Check sheet for the modelled part. Datum: model origin and axes. Units: mm. Round coordinates to 2 decimals unless told otherwise and drop trailing zeros. Order: outer loops, then holes, each group sorted by start corner. A loop starts at its lowest first (then second) coordinate and runs counter-clockwise, first axis right, second up. Notation, with made-up numbers: (-17, 42.5) -> (37, 42.5) arc R17 cw to (37, 65.5) -> close; hole circle Ø9 at (7, 5). An arc over 180 degrees is marked (long way). Answer in a Markdown table with one row per item. Add a question column.
1. Depth check by flat-ended pin: P1, Ø1.9, axis at x = 1, z = 76.5, coming from the -Y side. Enter the tip coordinate at first touch or a pass-through.
2. Sectioned sample at D-D, the plane z = 27. Record the boundary of the cut face in (x, y).
3. Sectioned sample at B-B, the plane x = 24.8. Record the boundary of the cut face in (y, z), then the cut area to 3 significant figures.
4. Sectioned sample at A-A, the plane z = 0. Record the boundary of the cut face in (x, y), then the cut area to 3 significant figures.
5. Sectioned sample at C-C, the plane y = 3. Count the separate pieces of the cut face and the enclosed holes in it, then the cut area to 3 significant figures.
6. Material ranges on L1, parallel to Z at x = 0, y = 2.6; L2, parallel to X at y = 1.15, z = 24.8; L3, parallel to Y at x = 22.5, z = 75.5, recorded low to high. Write a range as from..to.
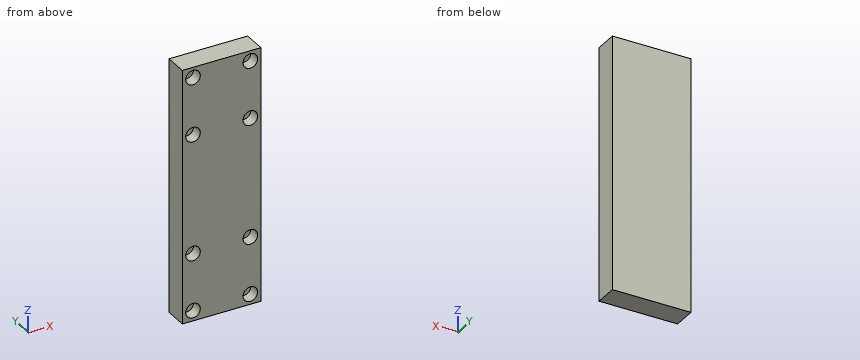
```python
from build123d import *

# Parameters (mm, degrees)
SKETCH2_W           = 34
SKETCH2_H           = 55
BOSS_EXTRUDE1_DEPTH = 10
SKETCH1_R           = 3.15
CUT_EXTRUDE1_DEPTH  = 5


with BuildPart() as part:
    # Sketch2 → Boss-Extrude1 (new body)
    with BuildSketch(Plane(origin=(0, 0, 0), x_dir=(1, 0, 0), z_dir=(0, 1, 0))):
        with Locations((12.4, -23.06737043)):
            Rectangle(SKETCH2_W, SKETCH2_H)
    extrude(amount=BOSS_EXTRUDE1_DEPTH)

    # Sketch1 → Cut-Extrude1 (cut)
    with BuildSketch(Plane(origin=(0, 0, 0), x_dir=(1, 0, 0), z_dir=(0, 1, 0))):
        Circle(SKETCH1_R)
        with Locations((24.8, 0)):
            Circle(SKETCH1_R)
        with Locations((0, -24.8)):
            Circle(SKETCH1_R)
        with Locations((24.8, -24.8)):
            Circle(SKETCH1_R)
    extrude(amount=CUT_EXTRUDE1_DEPTH, mode=Mode.SUBTRACT)

    # Mirror1: part across plane


with BuildPart() as part_1:
    add(part.part)
    add(part.part.mirror(Plane(origin=(-4.6, 10, 50.56737043), x_dir=(1, 0, 0), z_dir=(0, 0, -1))))


solid = part_1.part
```
Answer key:
| question | item | result |
|---|---|---|
| 1 | P1 | stops at y = 5 |
| 2 | outline | (-4.6, 0) -> (-2.25, 0) -> (-2.25, 5) -> (2.25, 5) -> (2.25, 0) -> (22.55, 0) -> (22.55, 5) -> (27.05, 5) -> (27.05, 0) -> (29.4, 0) -> (29.4, 10) -> (-4.6, 10) -> close |
| 3 | outline | (0, -4.43) -> (10, -4.43) -> (10, 105.57) -> (0, 105.57) -> (0, 104.28) -> (5, 104.28) -> (5, 97.98) -> (0, 97.98) -> (0, 79.48) -> (5, 79.48) -> (5, 73.18) -> (0, 73.18) -> (0, 27.95) -> (5, 27.95) -> (5, 21.65) -> (0, 21.65) -> (0, 3.15) -> (5, 3.15) -> (5, -3.15) -> (0, -3.15) -> close |
| 3 | area | 974 mm² |
| 4 | outline | (-4.6, 0) -> (-3.15, 0) -> (-3.15, 5) -> (3.15, 5) -> (3.15, 0) -> (21.65, 0) -> (21.65, 5) -> (27.95, 5) -> (27.95, 0) -> (29.4, 0) -> (29.4, 10) -> (-4.6, 10) -> close |
| 4 | area | 277 mm² |
| 5 | separate pieces | 1 |
| 5 | enclosed holes | 8 |
| 5 | area | 3,490 mm² |
| 6 | L1 | z = -4.43..-3.15, 3.15..21.65, 27.95..73.18, 79.48..97.98, 104.28..105.57 |
| 6 | L2 | x = -4.6..-3.15, 3.15..21.65, 27.95..29.4 |
| 6 | L3 | y = 5..10 |
